```python
from build123d import *

# Parameters (mm, degrees)
F1_DEPTH = 10
F2_R     = 3


with BuildPart() as f1:
    # F0 (on Right) → F1 (new body)
    with BuildSketch(Plane.YZ):
        Polygon((50, 0), (0, 0), (-50, 0), (-50, -165), (-42.5, -165), (-42.5, -163.5), (-45, -163.5), (-45, -157.5), (-41, -157.5), (-41, -153.5), (-45, -153.5), (-45, -5), (0, -5), (45, -5), (45, -153.5), (41, -153.5), (41, -157.5), (45, -157.5), (45, -163.5), (42.5, -163.5), (42.5, -165), (50, -165), align=None)
    extrude(amount=F1_DEPTH)

    # F2
    f2_edges = [f1.edges().sort_by_distance(p)[0] for p in [
        (5, -45, -5),
        (5, 45, -5),
        (5, 45, -153.5),
        (5, -45, -153.5),
    ]]
    fillet(f2_edges, radius=F2_R)


solid = f1.part
```
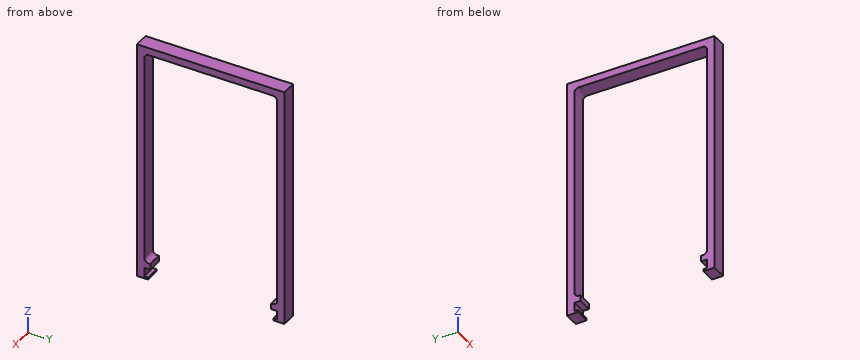
Work out the finished part from the listing and answer in its coordinate system (mm). Round coordinates to 2 decimals unless told otherwise and drop trailing zeros. Order: outer loops, then holes, each group sorted by start corner. A loop starts at its lowest first (then second) coordinate and runs counter-clockwise, first axis right, second up.
Q1. A cutting plane is placed at C-C, the plane y = -8. Determine the outline of the cut face in (x, z), then the cut area to 3 significant figures.
Solution:
outline: (0, -5) - (10, -5) - (10, 0) - (0, 0) - close
area: 50.0 mm2
Q2. Given pin 1 Ø6 at (x, y) = (2, -20) entering from +Z; pin 2 Ø5 at (x, y) = (6.5, 7.5) entering from -Z, each flat-ended and moving along its own axis, determine where each tip first touches the part or whether it passes through.
Solution:
pin 1: stops at z = 0
pin 2: stops at z = -5
Q3. A cutting plane is placed at B-B, the plane x = 6.25. Determine the outline of the cut face in (y, z).
Solution:
outline: (-50, -165) - (-42.5, -165) - (-42.5, -163.5) - (-45, -163.5) - (-45, -157.5) - (-41, -157.5) - (-41, -153.5) - (-42, -153.5) arc R3 cw to (-45, -150.5) - (-45, -8) arc R3 cw to (-42, -5) - (42, -5) arc R3 cw to (45, -8) - (45, -150.5) arc R3 cw to (42, -153.5) - (41, -153.5) - (41, -157.5) - (45, -157.5) - (45, -163.5) - (42.5, -163.5) - (42.5, -165) - (50, -165) - (50, 0) - (-50, 0) - close
Q4. Find the intervals of material crossed by line 1 along Y through (x, z) = (4.5, -10); line 2 along Z through (x, y) = (6.5, 44.5); line 3 along Z through (x, y) = (8, -38.5), in increasing order.
Solution:
line 1: y = -50 to -45, 45 to 50
line 2: z = -165 to -163.5, -157.5 to -152.16, -6.34 to 0
line 3: z = -5 to 0
Q5. A cutting plane is placed at A-A, the plane z = -50.5. Determine the outline of the cut face in (x, y), then the cut area to 3 significant figures.
Solution:
outline: (0, -50) - (10, -50) - (10, -45) - (0, -45) - close; (0, 45) - (10, 45) - (10, 50) - (0, 50) - close
area: 100 mm2
